Source: CAD feature listing. Evaluate the final solid. Frame: model axes, mm. Coordinates: 2 decimals unless noted, no trailing zeros. Loops run counter-clockwise (first coordinate to the right, second up) from the corner with the lowest first, then second, coordinate; pieces in that order, holes last.
```python
from build123d import *

# Parameters (mm, degrees)
BOSS_EXTRUDE1_DEPTH = 1
SKETCH2_R           = 3.5
CUT_EXTRUDE1_DEPTH  = 81.498297773
SKETCH3_R           = 45
CUT_EXTRUDE2_DEPTH  = 81.498297773


with BuildPart() as part:
    # Sketch1 → Boss-Extrude1 (new body)
    with BuildSketch(Plane(origin=(0, 0, 0), x_dir=(1, 0, 0), z_dir=(0, 1, 0))):
        with BuildLine():
            Line((2, -60.044427996), (51, -31.754264805))
            ThreePointArc((51, -31.754264805), (52.464101615, -30.29016319), (53, -28.29016319))
            Line((53, -28.29016319), (53, 28.29016319))
            ThreePointArc((53, 28.29016319), (52.464101615, 30.29016319), (51, 31.754264805))
            Line((51, 31.754264805), (2, 60.044427996))
            ThreePointArc((2, 60.044427996), (0, 60.580326381), (-2, 60.044427996))
            Line((-2, 60.044427996), (-51, 31.754264805))
            ThreePointArc((-51, 31.754264805), (-52.464101615, 30.29016319), (-53, 28.29016319))
            Line((-53, 28.29016319), (-53, -28.29016319))
            ThreePointArc((-53, -28.29016319), (-52.464101615, -30.29016319), (-51, -31.754264805))
            Line((-51, -31.754264805), (-2, -60.044427996))
            ThreePointArc((-2, -60.044427996), (0, -60.580326381), (2, -60.044427996))
        make_face()
    extrude(amount=BOSS_EXTRUDE1_DEPTH)

    # Sketch2 → Cut-Extrude1 (cut, through all)
    with BuildSketch(Plane(origin=(0, 1, 0), x_dir=(1, 0, 0), z_dir=(0, 1, 0))):
        with Locations(Location((0, 51, 0), (0, 0, 270))):
            Circle(SKETCH2_R)
        with Locations(Location((44.167295593, 25.5, 0), (0, 0, 270))):
            Circle(SKETCH2_R)
        with Locations(Location((44.167295593, -25.5, 0), (0, 0, 270))):
            Circle(SKETCH2_R)
        with Locations(Location((0, -51, 0), (0, 0, 270))):
            Circle(SKETCH2_R)
        with Locations(Location((-44.167295593, -25.5, 0), (0, 0, 270))):
            Circle(SKETCH2_R)
        with Locations(Location((-44.167295593, 25.5, 0), (0, 0, 270))):
            Circle(SKETCH2_R)
    extrude(amount=-CUT_EXTRUDE1_DEPTH, mode=Mode.SUBTRACT)

    # Sketch3 → Cut-Extrude2 (cut, through all)
    with BuildSketch(Plane.XZ):
        with Locations(Location((0, 0, 0), (0, 0, 270))):
            Circle(SKETCH3_R)
    extrude(amount=-CUT_EXTRUDE2_DEPTH, mode=Mode.SUBTRACT)


solid = part.part
```
Q1. Draft query along Z for faces 1 (the cylindrical face through (45.22, 0.51, 28.84)), 2 (the flat face through (-26.157, 0.493, -46.097)), 3 (the cylindrical face through (-17.235, 0.493, -41.569)), 4 (the flat face through (-26.843, 0.493, 45.701)). Return one class per face: released by +Z, released by -Z, zero draft, split by the parting line, or undercut.
Q2. Material intervals for line 1 along X through (y, z) = (0.35, 28); line 2 along Z through (x, y) = (47, 0.7); line 3 along Z through (x, y) = (34, 0.75), sorted ascending.
Q3. Section query B-B on x = 0. Return the cut outline in (y, z), then the cut area to 3 significant figures.
Q4. Section query A-A on z = 0. Return the cut outline in (x, y).
Q5. Section query C-C on x = -19.5. Return the cut outline in (y, z), then the cut area to 3 significant figures.
Q6. First-contact query: pin 1 Ø6.5 at (x, z) = (-44.17, -25.5) entering from +Y. Flat tip, straight axial feed; report the tip coordinate or a pass-through.
Q7. Section query D-D on y = 0.7. Return the cut outline in (x, z), then the cut area to 3 significant figures.
Resolved:
1. face 1: undercut
1. face 2: released by -Z
1. face 3: undercut
1. face 4: released by +Z
2. line 1: x = -53 to -46.62, -41.72 to -35.23, 35.23 to 41.72, 46.62 to 53
2. line 2: z = -34.06 to -27.56, -23.44 to 23.44, 27.56 to 34.06
2. line 3: z = -41.57 to -29.48, 29.48 to 41.57
3. outline: (0, -60.58) - (1, -60.58) - (1, -54.5) - (0, -54.5) - close; (0, -47.5) - (1, -47.5) - (1, -45) - (0, -45) - close; (0, 45) - (1, 45) - (1, 47.5) - (0, 47.5) - close; (0, 54.5) - (1, 54.5) - (1, 60.58) - (0, 60.58) - close
3. area: 17.2 mm2
4. outline: (-53, 0) - (-45, 0) - (-45, 1) - (-53, 1) - close; (45, 0) - (53, 0) - (53, 1) - (45, 1) - close
5. outline: (0, -49.94) - (1, -49.94) - (1, -40.56) - (0, -40.56) - close; (0, 40.56) - (1, 40.56) - (1, 49.94) - (0, 49.94) - close
5. area: 18.8 mm2
6. pin 1: passes through
7. outline: (-53, -28.29) arc R4 ccw to (-51, -31.75) - (-2, -60.04) arc R4 ccw to (2, -60.04) - (51, -31.75) arc R4 ccw to (53, -28.29) - (53, 28.29) arc R4 ccw to (51, 31.75) - (2, 60.04) arc R4 ccw to (-2, 60.04) - (-51, 31.75) arc R4 ccw to (-53, 28.29) - close; hole circle Ø7 at (-44.17, -25.5); hole circle Ø7 at (-44.17, 25.5); hole circle Ø90 at (0, 0); hole circle Ø7 at (0, -51); hole circle Ø7 at (0, 51); hole circle Ø7 at (44.17, -25.5); hole circle Ø7 at (44.17, 25.5)
7. area: 3,130 mm2
